```python
from build123d import *

# Parameters (mm, degrees)
SKETCH3_R          = 17
CUT_EXTRUDE1_DEPTH = 10
SKETCH4_R          = 3
CUT_EXTRUDE2_DEPTH = 28


with BuildPart() as part:
    # Sketch2 → Revolve1 (revolve)
    with BuildSketch(Plane.XY, mode=Mode.PRIVATE) as revolve1_sk:
        Polygon((0, 0), (0, 40), (2, 40), (2, 27), (8, 27), (8, 0), align=None)
    revolve(revolve1_sk.sketch.rotate(Axis((8, 0, 0), (-1, 0, 0)), 90), axis=Axis((8, 0, 0), (-1, 0, 0)))

    # Sketch3 → Cut-Extrude1 (cut)
    with BuildSketch(Plane(origin=(8, 0, 0), x_dir=(0, 0, -1), z_dir=(1, 0, 0))):
        Circle(SKETCH3_R)
    extrude(amount=-CUT_EXTRUDE1_DEPTH, mode=Mode.SUBTRACT)

    # Sketch4 → Cut-Extrude2 (cut)
    with BuildSketch(Plane(origin=(8, 0, 0), x_dir=(0, 0, -1), z_dir=(1, 0, 0))):
        with Locations((0, -32.5)):
            Circle(SKETCH4_R)
        with Locations((32.5, 0)):
            Circle(SKETCH4_R)
        with Locations((0, 32.5)):
            Circle(SKETCH4_R)
        with Locations((-32.5, 0)):
            Circle(SKETCH4_R)
    extrude(amount=-CUT_EXTRUDE2_DEPTH, mode=Mode.SUBTRACT)


solid = part.part
```
Can you work these out from the model? Positions are in its coordinate system, mm. A direction names the side the tool comes from. Coordinates: 2 decimals unless noted, no trailing zeros. Loops run counter-clockwise (first coordinate to the right, second up) from the corner with the lowest first, then second, coordinate; pieces in that order, holes last. Notation, with made-up numbers: (88.5, 70.5) - (120.5, 70.5) arc R26 ccw to (120.5, 102.5) - close; hole circle Ø10 at (31.25, -23.5). An arc over 180 degrees is marked (long way). Answer as CSV lines item,"result". Start each with the question number.
1) Thinking about a two-plate mould opening in Z: for faces 1 (the cylindrical face through (1.01, 34.53, 2.21)), 2 (the flat face through (0, -0.6, 17.2)), 3 (the cylindrical face through (1.01, -1.76, 39.96)), 4 (the cylindrical face through (1, 0.1, 35.5)), which applies, pulls with the +Z half, pulls with the -Z half, needs draft (parallel to the pull), parting line crosses it, or undercut?
2) Suppose I cut it at A-A (z = 0). Please give me the cut outline in (x, y), plus the area to 3 significant figures.
3) I need wall thicknesses on line 1 (Y direction, x = 0.8, z = 0); line 2 (Y direction, x = 2.75, z = 0); line 3 (Y direction, x = 6, z = 4). Which ranges of each line are inside material? Lowest first, please. Write a range as from..to.
4) For pin 1 (3 mm diameter, centred on x = 5.5, y = -8, fed in from +Z); pin 2 (1.5 mm diameter, centred on x = 4.5, z = 22, fed in from -Y); pin 3 (1.5 mm diameter, centred on x = 1.5, y = -29, fed in from +Z), each with a flat end and sliding along its axis, tell me the tip position at first contact or that it passes through.
5) Suppose I cut it at C-C (z = 32.5). Please give me the cut outline in (x, y), plus the area to 3 significant figures.
6) Which directions (+Z, -Z, +X, -X, +Y, -Y) give clear straight access to the entire face, cutting with the end or side of a thin tool? Please do faces 5 (the cylindrical face through (1, 0.1, -29.5)), 6 (the flat face through (2, -27.2, 0.6)).
Check result:
1,face 1,"undercut"
1,face 2,"needs draft"
1,face 3,"parting line crosses it"
1,face 4,"undercut"
2,outline,"(0, -40) - (2, -40) - (2, -35.5) - (0, -35.5) - close; (0, -29.5) - (2, -29.5) - (2, -27) - (8, -27) - (8, -17) - (0, -17) - close; (0, 17) - (8, 17) - (8, 27) - (2, 27) - (2, 29.5) - (0, 29.5) - close; (0, 35.5) - (2, 35.5) - (2, 40) - (0, 40) - close"
2,area,"188 mm²"
3,line 1,"y = -40..-35.5, -29.5..-17, 17..29.5, 35.5..40"
3,line 2,"y = -27..-17, 17..27"
3,line 3,"y = -26.7..-16.52, 16.52..26.7"
4,pin 1,"stops at z = 26.21"
4,pin 2,"stops at y = -16.66"
4,pin 3,"stops at z = 28.32"
5,outline,"(0, -23.32) - (2, -23.32) - (2, -3) - (0, -3) - close; (0, 3) - (2, 3) - (2, 23.32) - (0, 23.32) - close"
5,area,"81.3 mm²"
6,face 5,"+X, -X"
6,face 6,"+X"
